Design review of the part shown in the three views and the two pictorial views. Dimensions are in mm from the part's minimum x, y and z. A direction names the side the tool comes from. Coordinates: 2 decimals unless noted, no trailing zeros. Loops run counter-clockwise (first coordinate to the right, second up) from the corner with the lowest first, then second, coordinate; pieces in that order, holes last. Notation, with made-up numbers: M 46.5,78 L 54.5,78 A4 ccw 54.5,83 Z; hole C 51,81.5 d4. An arc over 180 degrees is marked long. Answer as a JSON object with one key per item and string values. Group by question number.
Item 1: Tool access review of the marked faces 4 and 5: name each direction out of +Z, -Z, +X, -X, +Y, -Y from which nothing blocks a thin tool from reaching the whole face with its end or side.
Item 2: Wall thickness on L1, parallel to Y at x = 29, z = 4.5 (1 decimal); L2, parallel to X at y = 3.5, z = 24 (1 decimal); L3, parallel to Z at x = 37, y = 45: over which ranges is each line inside the solid? List them lowest first. Write a range as from..to.
Item 3: Add section A-A (z = 58.5). State the section outline as (x, y) points (1 decimal), then the cut area to 3 significant figures.
Item 4: Mouldability with a two-part tool opening along Y and no side actions: class the marked faces 1, 2 and 3 as +Y half, -Y half, draft (parallel to the pull), parting line (faces both ways), or undercut.
Item 5: Add section B-B (z = 9). State the section outline as (x, y) points (1 decimal), then the cut area to 3 significant figures.
Item 6: Insertion check: pin 1 (17 mm diameter, centred on x = 26.99, y = 26.99, fed in from +Z); pin 2 (1.5 mm diameter, centred on y = 7, z = 12.5, fed in from +X) (1 decimal); pin 3 (12 mm diameter, centred on x = 31.5, z = 66.5, fed in from -Y); pin 4 (4 mm diameter, centred on x = 14.5, z = 15, fed in from +Y) (1 decimal). Each pin has a flat end and moves straight along its axis. Give the tip position at first contact, or say it passes through.
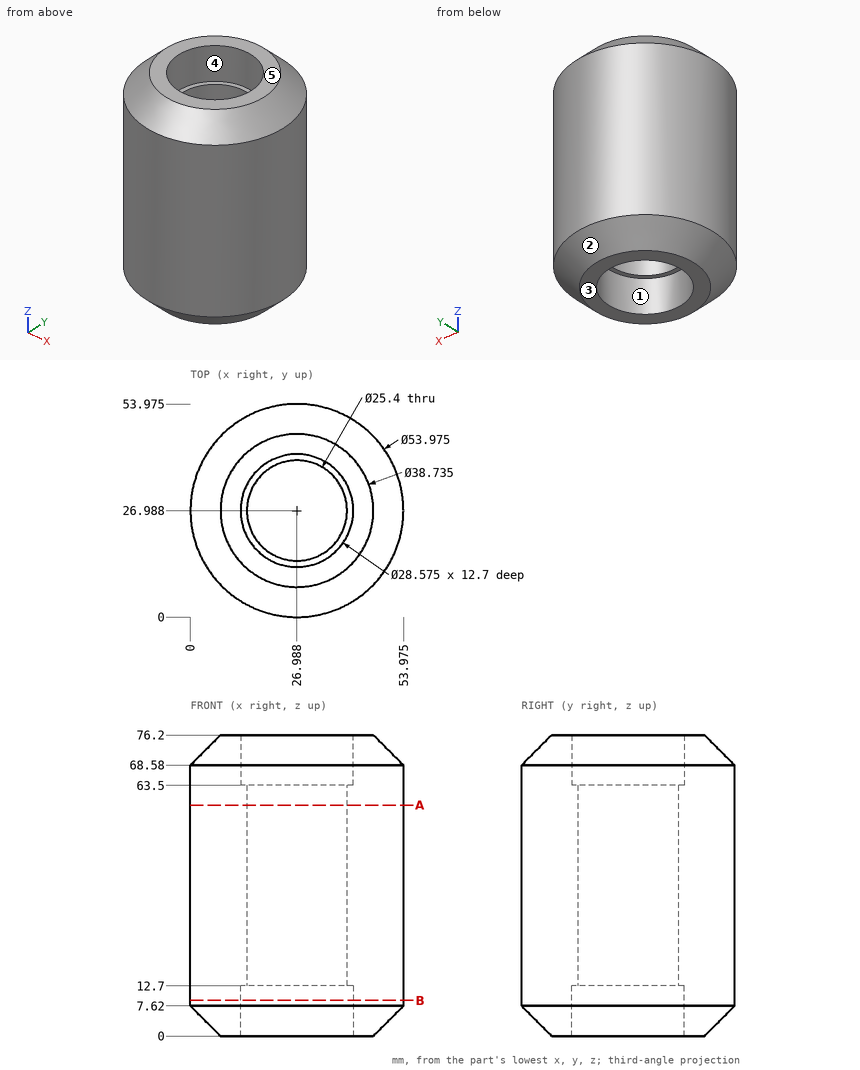
From the geometry:
{
 "1": {"face 4": "+Z", "face 5": "+Z, +X, -X, +Y, -Y"},
 "2": {"L1": "y = 3.2..12.8, 41.1..50.8", "L2": "x = 13.7..40.3", "L3": "z = 1.24..74.96"},
 "3": {"outline": "C 27,27 d54; hole C 27,27 d25.4", "area": "1,780 mm²"},
 "4": {"face 1": "undercut", "face 2": "parting line", "face 3": "draft"},
 "5": {"outline": "C 27,27 d54; hole C 27,27 d28.6", "area": "1,650 mm²"},
 "6": {"pin 1": "passes through", "pin 2": "stops at x = 45.9", "pin 3": "stops at y = 0", "pin 4": "stops at y = 51.9"}
}
